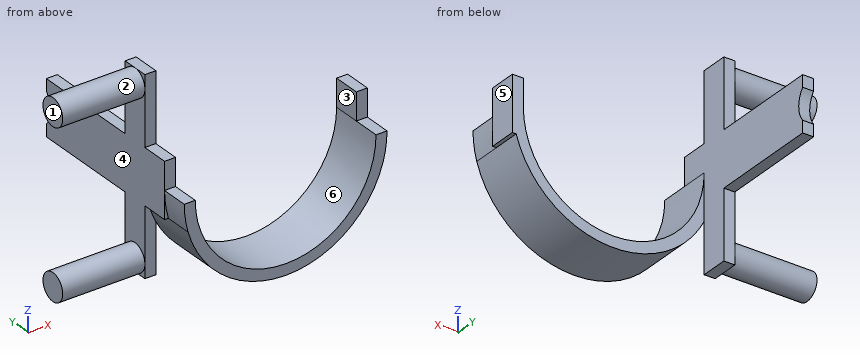
from build123d import *

# Parameters (mm, degrees)
EXTRUDE_1_DEPTH     = 40
SKETCH_2_W          = 8
SKETCH_2_H          = 40
EXTRUDE_2_DEPTH     = 100
SKETCH_3_R          = 18
CUT_EXTRUDE_1_DEPTH = 149
SKETCH_5_W          = 87.00766185
SKETCH_5_H          = 115.01495327
CUT_EXTRUDE_2_DEPTH = 10
SKETCH_6_R          = 85.063361003
CUT_EXTRUDE_3_DEPTH = 20
SKETCH_7_W          = 140
SKETCH_7_H          = 20
EXTRUDE_3_DEPTH     = 8
SKETCH_9_R          = 10
EXTRUDE_4_DEPTH     = 60


with BuildPart() as part:
    # 草图1 → 凸台-拉伸1 (new body)
    with BuildSketch(Plane(origin=(0, 0, 0), x_dir=(1, 0, 0), z_dir=(0, 1, 0))):
        with BuildLine():
            Line((-74, 20), (-71.246052522, 20))
            ThreePointArc((-71.246052522, 20), (0, 74), (71.246052522, 20))
            Line((71.246052522, 20), (74, 20))
            Line((74, 20), (74, -20))
            Line((74, -20), (66, -20))
            Line((66, -20), (66, 0))
            ThreePointArc((66, 0), (0, 66), (-66, 0))
            Line((-66, 0), (-66, -20))
            Line((-66, -20), (-74, -20))
            Line((-74, -20), (-74, 20))
        make_face()
    extrude(amount=EXTRUDE_1_DEPTH)

    # 草图2 → 凸台-拉伸2 (add)
    with BuildSketch(Plane(origin=(0, 40, 0), x_dir=(1, 0, 0), z_dir=(0, 1, 0))):
        with Locations((-70, 0)):
            Rectangle(SKETCH_2_W, SKETCH_2_H)
        with Locations((70, 0)):
            Rectangle(SKETCH_2_W, SKETCH_2_H)
    extrude(amount=EXTRUDE_2_DEPTH)

    # 草图3 → 切除-拉伸1 (cut, through all)
    with BuildSketch(Plane.ZY.offset(74)):
        with Locations((0, 154)):
            Circle(SKETCH_3_R)
    extrude(amount=-CUT_EXTRUDE_1_DEPTH, mode=Mode.SUBTRACT)

    # 草图5 → 切除-拉伸2 (cut)
    with BuildSketch(Plane(origin=(74, 0, 0), x_dir=(0, 0, -1), z_dir=(1, 0, 0))):
        with Locations((-23.503830925, 97.507476635)):
            Rectangle(SKETCH_5_W, SKETCH_5_H)
    extrude(amount=-CUT_EXTRUDE_2_DEPTH, mode=Mode.SUBTRACT)

    # 草图6 → 切除-拉伸3 (cut)
    with BuildSketch(Plane.XZ):
        Circle(SKETCH_6_R)
        with BuildLine():
            Line((-71.246052522, 20), (-66, 20))
            Line((-66, 20), (-66, 0))
            Line((-66, 0), (-74, 0))
            ThreePointArc((-74, 0), (0, -74), (74, 0))
            Line((74, 0), (66, 0))
            Line((66, 0), (66, 20))
            Line((66, 20), (71.246052522, 20))
            ThreePointArc((71.246052522, 20), (0, 74), (-71.246052522, 20))
        make_face(mode=Mode.SUBTRACT)
    extrude(amount=-CUT_EXTRUDE_3_DEPTH, mode=Mode.SUBTRACT)

    # 草图7 → 凸台-拉伸3 (add)
    with BuildSketch(Plane.ZY.offset(74)):
        with Locations((0, 50)):
            Rectangle(SKETCH_7_W, SKETCH_7_H)
    extrude(amount=-EXTRUDE_3_DEPTH)

    # 草图9 → 凸台-拉伸4 (add)
    with BuildSketch(Plane.ZY.offset(74)):
        with Locations((-60, 50)):
            Circle(SKETCH_9_R)
        with Locations((60, 50)):
            Circle(SKETCH_9_R)
    extrude(amount=EXTRUDE_4_DEPTH)


solid = part.part
Could you check a few things on this model? Use its own coordinates, in mm. Face numbers are marked on the shaded views. A direction names the side the tool comes from. Give positions to 0.01 mm unless a question says otherwise; leave off trailing zeros. Order: outer loops, then holes, each group sorted by start corner. A loop starts at its lowest first (then second) coordinate and runs counter-clockwise, first axis right, second up. Notation, with made-up numbers: (-16.5, 69) - (-1.5, 69) arc R31 cw to (-1.5, 103) - close; hole circle Ø6 at (-26, 83). An arc over 180 degrees is marked (long way). One line per item, written item: value. Start each with the question number.
1. Imagine slicing it at B-B on y = 32.5. List the corners of the cut face in (x, z) for me, plus the area to 3 significant figures.
2. Imagine slicing it at C-C on z = -38. List the corners of the cut face in (x, y) for me.
3. Imagine slicing it at A-A on z = 7. List the corners of the cut face in (x, y) for me.
4. If I drill on probe 1 along Z at (x, y) = (-100, 51); probe 2 along X at (y, z) = (115, 5); probe 3 along Z at (x, y) = (-68, 61.5), over which ranges is the centre line in solid material (lowest first)?
5. Thinking about a two-plate mould opening in Z: for the marked faces 4, 5 and 6, which applies, +Z half, -Z half, draft (parallel to the pull), parting line (faces both ways), or undercut?
6. For P1, Ø3, axis at x = -72.5, z = -14, coming from the -Y side; P2, Ø2, axis at x = 72.5, y = 34.5, coming from the -Z side; P3, Ø9, axis at x = -70, y = 117, coming from the +Z side; P4, Ø9, axis at x = -69.5, y = 11, coming from the +Z side, each with a flat end and sliding along its axis, tell me the tip position at first contact or that it passes through.
7. For the marked faces 1, 2 and 3, which set-ups out of +Z, -Z, +X, -X, +Y, -Y let a thin tool reach every point of the face, with its end or its side?
8. Imagine slicing it at D-D on x = -100. List the corners of the cut face in (y, z) for me, plus the area to 3 significant figures.
Values:
1. outline: (-74, -20) - (-71.25, -20) arc R74 ccw to (71.25, -20) - (74, -20) - (74, 20) - (66, 20) - (66, 0) arc R66 cw to (-66, 0) - (-66, 20) - (-74, 20) - close
1. area: 2,120 mm²
2. outline: (-74, 40) - (-66, 40) - (-66, 60) - (-74, 60) - close; (-63.5, 0) - (-53.96, 0) - (-53.96, 40) - (-63.5, 40) - close; (53.96, 0) - (63.5, 0) - (63.5, 40) - (53.96, 40) - close
3. outline: (-74, 20) - (-66, 20) - (-66, 137.42) - (-74, 137.42) - close; (66, 20) - (74, 20) - (74, 40) - (66, 40) - close
4. probe 1: -69.95 to -50.05, 50.05 to 69.95
4. probe 2: -74 to -66
4. probe 3: -20 to 20
5. face 4: undercut
5. face 5: draft
5. face 6: +Z half
6. P1: y = 0
6. P2: z = -20
6. P3: z = 20
6. P4: z = 0
7. face 1: +Z, -Z, -X, +Y, -Y
7. face 2: -X
7. face 3: +Z, +Y, -Y
8. outline: circle Ø20 at (50, -60); circle Ø20 at (50, 60)
8. area: 628 mm²
